from build123d import *

# Parameters (mm, degrees)
SKETCH2_R           = 6
BOSS_EXTRUDE2_DEPTH = 16


with BuildPart() as part:
    # Sketch2 → Boss-Extrude2 (new body)
    with BuildSketch(Plane(origin=(0, 0, 0), x_dir=(1, 0, 0), z_dir=(0, 1, 0))):
        with BuildLine():
            Line((-15.25, -19), (-30.5, -19))
            Line((-30.5, -19), (-30.5, -13))
            Line((-30.5, -13), (-20.524290918, -13))
            Line((-20.524290918, -13), (-19, 0))
            ThreePointArc((-19, 0), (0, 19), (19, 0))
            Line((19, 0), (20.524290918, -13))
            Line((20.524290918, -13), (30.5, -13))
            Line((30.5, -13), (30.5, -19))
            Line((30.5, -19), (15.25, -19))
            Line((15.25, -19), (11.892967086, -14.817467189))
            ThreePointArc((11.892967086, -14.817467189), (0, -19), (-11.892967086, -14.817467189))
            Line((-11.892967086, -14.817467189), (-15.25, -19))
        make_face()
        Circle(SKETCH2_R, mode=Mode.SUBTRACT)
    extrude(amount=BOSS_EXTRUDE2_DEPTH)


solid = part.part
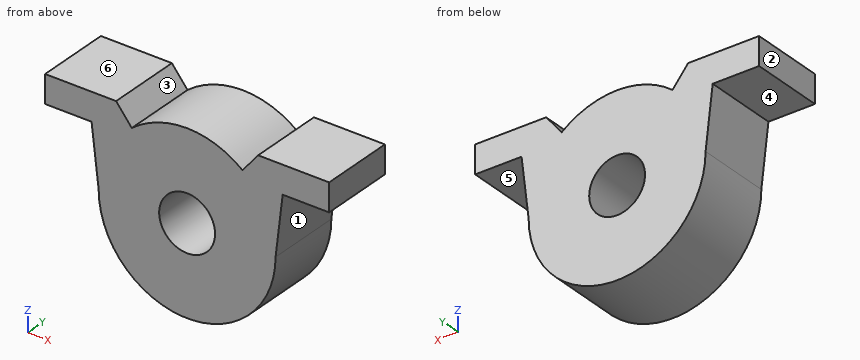
Verification items for the finished model (mm, model axes). Face numbers are marked on the shaded views. A direction names the side the tool comes from. Give positions to 0.01 mm unless a question says otherwise; leave off trailing zeros. Write each loop counter-clockwise with the first axis right and the second up, starting at its lowest first coordinate (ties: lowest second). Pieces come first, ordered by that corner, then holes.
(1) Gauge pin test, flat ends, axial feed: pin 1 (6 mm diameter, centred on y = 5, z = -12.5, fed in from -X); pin 2 (8 mm diameter, centred on x = -26, y = 8.5, fed in from -Z); pin 3 (10 mm diameter, centred on x = -1.5, z = -2, fed in from -Y); pin 4 (1 mm diameter, centred on y = 8, z = -1, fed in from +X). Record the tip position at first contact, or that the pin passes through.
(2) Access from +Z, -Z, +X, -X, +Y, -Y to the whole of each face (thin tool, end or side, straight path). Record for the marked faces 4, 5 and 6.
(3) Mould release check, pull along X, two halves, no side actions. Record for the marked faces 1, 2 and 3: +X half, -X half, draft (parallel to the pull), parting line (faces both ways), or undercut.
(4) Material ranges on line 1 (X direction, y = 10, z = 0); line 2 (X direction, y = 5, z = 17); line 3 (Z direction, x = -26, y = 4.5), recorded low to high.
(5) Cross-section at B-B (y = 4.25). Enter the section's corners in (x, z), plus the area to 3 significant figures.
(6) Cross-section at A-A (x = 2). Enter the section's corners in (y, z).
(7) Cross-section at C-C (z = 15.5). Enter the section's corners in (x, y), plus the area to 3 significant figures.
(8) Cross-section at D-D (z = 3.5). Enter the section's corners in (x, y).
Worked out:
1. pin 1: stops at x = -16.45
1. pin 2: stops at z = 13
1. pin 3: stops at y = 0
1. pin 4: stops at x = 18.99
2. face 4: -Z, -X, +Y, -Y
2. face 5: -Z, +X, +Y, -Y
2. face 6: +Z, +X, -X, +Y, -Y
3. face 1: +X half
3. face 2: -X half
3. face 3: undercut
4. line 1: x = -19 to -6, 6 to 19
4. line 2: x = -30.5 to -13.64, -8.49 to 8.49, 13.64 to 30.5
4. line 3: z = 13 to 19
5. outline: (-30.5, 13) - (-20.52, 13) - (-19, 0) arc R19 ccw to (19, 0) - (20.52, 13) - (30.5, 13) - (30.5, 19) - (15.25, 19) - (11.89, 14.82) arc R19 ccw to (-11.89, 14.82) - (-15.25, 19) - (-30.5, 19) - close; hole circle Ø12 at (0, 0)
5. area: 1,290 mm2
6. outline: (0, -18.89) - (16, -18.89) - (16, -5.66) - (0, -5.66) - close; (0, 5.66) - (16, 5.66) - (16, 18.89) - (0, 18.89) - close
7. outline: (-30.5, 0) - (-12.44, 0) - (-12.44, 16) - (-30.5, 16) - close; (-10.99, 0) - (10.99, 0) - (10.99, 16) - (-10.99, 16) - close; (12.44, 0) - (30.5, 0) - (30.5, 16) - (12.44, 16) - close
7. area: 930 mm2
8. outline: (-19.41, 0) - (-4.87, 0) - (-4.87, 16) - (-19.41, 16) - close; (4.87, 0) - (19.41, 0) - (19.41, 16) - (4.87, 16) - close
